Can you work these out from the model? Positions are in its coordinate system, mm. Face numbers are marked on the shaded views. A direction names the side the tool comes from. Round coordinates to 2 decimals unless told otherwise and drop trailing zeros. Write each loop counter-clockwise with the first axis right and the second up, starting at its lowest first coordinate (ties: lowest second). Pieces come first, ordered by that corner, then holes. Notation, with made-up numbers: M 53,68 L 112,68 A13 ccw 112,88 Z; hole C -20,-11.5 d5. An arc over 180 degrees is marked long. Answer in a Markdown table with one row per item. Add a question column.
(1) Suppose I cut it at A-A, the plane x = 0. Write out the boundary of the cut face in (y, z).
(2) For the marked faces 3 and 4, which set-ups out of +Z, -Z, +X, -X, +Y, -Y let a thin tool reach every point of the face, with its end or its side?
(3) If I drill on probe 1 along Y at (x, z) = (0, 4.3); probe 2 along Z at (x, y) = (22, -19); probe 3 along Y at (x, z) = (0, 2.1), over which ranges is the centre line in solid material (lowest first)?
(4) I'm going to push flat-ended pins straight in: pin 1 (1.5 mm diameter, centred on x = -0.5, y = -3, fed in from -Z); pin 2 (4 mm diameter, centred on y = 15.5, z = 2, fed in from -X); pin 3 (3 mm diameter, centred on y = 7.5, z = 6, fed in from -X). Where does each tip first touch, or does it pass through?
(5) Suppose I cut it at D-D, the plane x = -24.5. Write out the boundary of the cut face in (y, z), then the cut area to 3 significant figures.
(6) Suppose I cut it at C-C, the plane y = 15. Write out the boundary of the cut face in (x, z).
(7) If we mould it in two halves opening along X, with no side actions, what happens to the marked faces 1 and 2? For each: released by +X, released by -X, zero draft, split by the parting line, or undercut.
from build123d import *

# Parameters (mm, degrees)
ESQUISSE1_R                  = 30
ESQUISSE1_R_2                = 11
BOSS_EXTRU_1_DEPTH           = 6
ESQUISSE2_R                  = 30
BOSS_EXTRU_2_DEPTH           = 2
ENL_V_MAT_EXTRU_1_DEPTH      = 1
ENL_V_MAT_EXTRU_1_DEPTH_BACK = 1
ESQUISSE3_R                  = 30
ESQUISSE3_R_2                = 29


with BuildPart() as part:
    # Esquisse1 → Boss.-Extru.1 (new body)
    with BuildSketch(Plane.XY):
        Circle(ESQUISSE1_R)
        Circle(ESQUISSE1_R_2, mode=Mode.SUBTRACT)
    extrude(amount=BOSS_EXTRU_1_DEPTH)

    # Esquisse2 → Boss.-Extru.2 (add)
    with BuildSketch(Plane.XY.offset(6)):
        Circle(ESQUISSE2_R)
    extrude(amount=BOSS_EXTRU_2_DEPTH)

    # Esquisse3 → Enlèv. mat.-Extru.1 (cut, two sides: drawn at the far end of the back side and taken through both)
    with BuildSketch(Plane.XY.offset(4).offset(-ENL_V_MAT_EXTRU_1_DEPTH_BACK)):
        Circle(ESQUISSE3_R)
        Circle(ESQUISSE3_R_2, mode=Mode.SUBTRACT)
    extrude(amount=ENL_V_MAT_EXTRU_1_DEPTH + ENL_V_MAT_EXTRU_1_DEPTH_BACK, mode=Mode.SUBTRACT)


solid = part.part
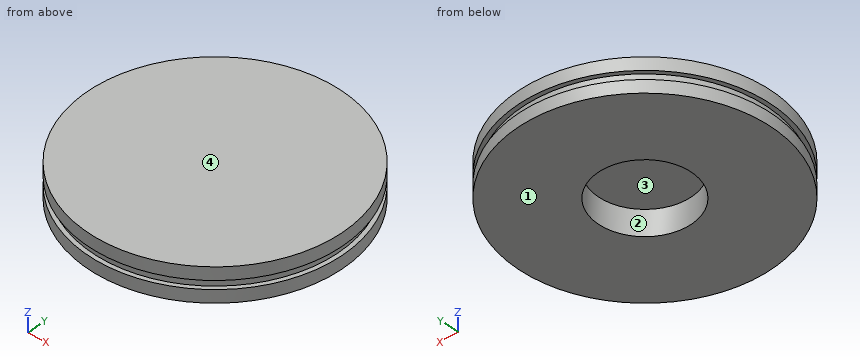
Calculated:
| question | item | result |
|---|---|---|
| 1 | outline | M -30,0 L -11,0 L -11,6 L 11,6 L 11,0 L 30,0 L 30,3 L 29,3 L 29,5 L 30,5 L 30,8 L -30,8 L -30,5 L -29,5 L -29,3 L -30,3 Z |
| 2 | face 3 | -Z |
| 2 | face 4 | +Z, +X, -X, +Y, -Y |
| 3 | probe 1 | -29 to -11, 11 to 29 |
| 3 | probe 2 | 0 to 3, 5 to 8 |
| 3 | probe 3 | -30 to -11, 11 to 30 |
| 4 | pin 1 | z = 6 |
| 4 | pin 2 | x = -26.79 |
| 4 | pin 3 | x = -29.39 |
| 5 | outline | M -17.31,0 L 17.31,0 L 17.31,3 L 15.52,3 L 15.52,5 L 17.31,5 L 17.31,8 L -17.31,8 L -17.31,5 L -15.52,5 L -15.52,3 L -17.31,3 Z |
| 5 | area | 270 mm² |
| 6 | outline | M -25.98,0 L 25.98,0 L 25.98,3 L 24.82,3 L 24.82,5 L 25.98,5 L 25.98,8 L -25.98,8 L -25.98,5 L -24.82,5 L -24.82,3 L -25.98,3 Z |
| 7 | face 1 | zero draft |
| 7 | face 2 | undercut |
